Design review of the part built by this model. Coordinates are the model's own, in mm. A direction names the side the tool comes from. Give positions to 0.01 mm unless a question says otherwise; leave off trailing zeros. Order: outer loops, then holes, each group sorted by start corner. A loop starts at its lowest first (then second) coordinate and runs counter-clockwise, first axis right, second up. Notation, with made-up numbers: (8, 7) -> (48, 7) arc R21 ccw to (48, 23) -> close; hole circle Ø1 at (61.5, -37). An arc over 180 degrees is marked (long way). Answer in a Markdown table with one row per item. Add a question column.
```python
from build123d import *

# Parameters (mm, degrees)
SKETCH1_W           = 7.25
SKETCH1_H           = 20
SKETCH1_R           = 6
BOSS_EXTRUDE1_DEPTH = 40
SKETCH2_W           = 42
SKETCH2_H           = 22
CUT_EXTRUDE1_DEPTH  = 25
SKETCH3_R           = 2
CUT_EXTRUDE2_DEPTH  = 12
SKETCH4_R           = 9.5
CUT_EXTRUDE3_DEPTH  = 5
SKETCH5_R           = 9.5
CUT_EXTRUDE4_DEPTH  = 6
SKETCH7_W           = 7
SKETCH7_H           = 2
SKETCH7_H_2         = 1.8
CUT_EXTRUDE5_DEPTH  = 2.4
BOSS_EXTRUDE2_REACH = 75.701
SKETCH9_R           = 13.5
SKETCH9_R_2         = 10.05
BOSS_EXTRUDE3_REACH = 50.701
SKETCH10_R          = 10.05
SKETCH11_R          = 1.9
CUT_EXTRUDE7_DEPTH  = 13.5


with BuildPart() as part:
    # Sketch1 → Boss-Extrude1 (new body)
    with BuildSketch(Plane(origin=(0, 0, 0), x_dir=(1, 0, 0), z_dir=(0, 1, 0))):
        with BuildLine():
            Line((-30.25, -10), (-37.5, -10))
            Line((-37.5, -10), (-37.5, 10))
            Line((-37.5, 10), (-30.25, 10))
            Line((-30.25, 10), (-18.466185313, 10))
            ThreePointArc((-18.466185313, 10), (-13.083157843, 16.426532831), (-5.61521172, 20.235350191))
            Line((-5.61521172, 20.235350191), (-42.5, 10))
            Line((-42.5, 10), (-42.5, -10))
            Line((-42.5, -10), (-5.61521172, -20.235350191))
            ThreePointArc((-5.61521172, -20.235350191), (-13.083157843, -16.426532831), (-18.466185313, -10))
            Line((-18.466185313, -10), (-30.25, -10))
        make_face()
        with Locations((-33.875, 0)):
            Rectangle(SKETCH1_W, SKETCH1_H)
        with BuildLine():
            ThreePointArc((-18.466185313, 10), (-21, 0), (-18.466185313, -10))
            Line((-18.466185313, -10), (9.75, -10))
            Line((9.75, -10), (9.75, 10))
            Line((9.75, 10), (-18.466185313, 10))
        make_face()
        Circle(SKETCH1_R, mode=Mode.SUBTRACT)
        with BuildLine():
            Line((-30.25, 10), (-30.25, -10))
            Line((-30.25, -10), (-18.466185313, -10))
            ThreePointArc((-18.466185313, -10), (-21, 0), (-18.466185313, 10))
            Line((-18.466185313, 10), (-30.25, 10))
        make_face()
        with BuildLine():
            Line((9.75, -10), (-18.466185313, -10))
            ThreePointArc((-18.466185313, -10), (-13.083157843, -16.426532831), (-5.61521172, -20.235350191))
            ThreePointArc((-5.61521172, -20.235350191), (12.709849603, -16.717048874), (21, 0))
            ThreePointArc((21, 0), (12.709849603, 16.717048874), (-5.61521172, 20.235350191))
            ThreePointArc((-5.61521172, 20.235350191), (-13.083157843, 16.426532831), (-18.466185313, 10))
            Line((-18.466185313, 10), (9.75, 10))
            Line((9.75, 10), (17, 10))
            Line((17, 10), (17, -10))
            Line((17, -10), (9.75, -10))
        make_face()
        with Locations((13.375, 0)):
            Rectangle(SKETCH1_W, SKETCH1_H)
    extrude(amount=BOSS_EXTRUDE1_DEPTH)

    # Sketch2 → Cut-Extrude1 (cut)
    with BuildSketch(Plane(origin=(0, 40, 0), x_dir=(1, 0, 0), z_dir=(0, 1, 0))):
        with Locations((-10, 0)):
            Rectangle(SKETCH2_W, SKETCH2_H)
    extrude(amount=-CUT_EXTRUDE1_DEPTH, mode=Mode.SUBTRACT)

    # Sketch3 → Cut-Extrude2 (cut)
    with BuildSketch(Plane(origin=(0, 40, 0), x_dir=(1, 0, 0), z_dir=(0, 1, 0))):
        with Locations((14.75, 5)):
            Circle(SKETCH3_R)
        with Locations((14.75, -5)):
            Circle(SKETCH3_R)
        with Locations((-34.75, 5)):
            Circle(SKETCH3_R)
        with Locations((-34.75, -5)):
            Circle(SKETCH3_R)
    extrude(amount=-CUT_EXTRUDE2_DEPTH, mode=Mode.SUBTRACT)

    # Sketch4 → Cut-Extrude3 (cut)
    with BuildSketch(Plane(origin=(0, 15, 0), x_dir=(1, 0, 0), z_dir=(0, 1, 0))):
        Circle(SKETCH4_R)
    extrude(amount=-CUT_EXTRUDE3_DEPTH, mode=Mode.SUBTRACT)

    # Sketch5 → Cut-Extrude4 (cut)
    with BuildSketch(Plane.XZ):
        Circle(SKETCH5_R)
    extrude(amount=-CUT_EXTRUDE4_DEPTH, mode=Mode.SUBTRACT)

    # Sketch7 → Cut-Extrude5 (cut)
    with BuildSketch(Plane(origin=(0, 40, 0), x_dir=(1, 0, 0), z_dir=(0, 1, 0))):
        with Locations((-34.5, 0)):
            Rectangle(SKETCH7_W, SKETCH7_H)
        with Locations((14.5, 0)):
            Rectangle(SKETCH7_W, SKETCH7_H_2)
    extrude(amount=-CUT_EXTRUDE5_DEPTH, mode=Mode.SUBTRACT)

    # Sketch9 → Boss-Extrude2 (add, up to next)
    with BuildSketch(Plane(origin=(-8.961867673, -4.60437291, 43.807681948), x_dir=(0, 0.994521895, 0.104528463), z_dir=(0.199367934, 0.102430023, -0.974556575)), mode=Mode.PRIVATE) as boss_extrude2_sk1:
        with Locations((22.005607966, -1.9070974)):
            Circle(SKETCH9_R)
        with Locations((22.005607966, -1.9070974)):
            Circle(SKETCH9_R_2, mode=Mode.SUBTRACT)
    boss_extrude2_tool1 = extrude(boss_extrude2_sk1.sketch, amount=BOSS_EXTRUDE2_REACH, mode=Mode.PRIVATE) - part.part
    add(boss_extrude2_tool1.solids().sort_by_distance((-10.83068, 4.27413, 44.358542))[0])

    # Sketch10 → Boss-Extrude3 (add, up to next)
    with BuildSketch(Plane(origin=(-3.977669313, -2.043622323, 19.443767584), x_dir=(0.979924705, -0.020839624, 0.198275776), z_dir=(-0.199367934, -0.102430023, 0.974556575)), mode=Mode.PRIVATE) as boss_extrude3_sk1:
        with Locations((-1.9070974, 22.005607966)):
            Circle(SKETCH10_R)
    boss_extrude3_tool1 = extrude(boss_extrude3_sk1.sketch, amount=-BOSS_EXTRUDE3_REACH, mode=Mode.PRIVATE) - part.part
    add(boss_extrude3_tool1.solids().sort_by_distance((-5.846481, 19.88118, 21.365849))[0])

    # Sketch11 → Cut-Extrude7 (cut, symmetric)
    with BuildSketch(Plane(origin=(-1.868811857, 0.039743192, -0.378131217), x_dir=(-0.199367934, -0.102430023, 0.974556575), z_dir=(-0.979924705, 0.020839624, -0.198275776))):
        with Locations((32.45139953, 22.005607966)):
            Circle(SKETCH11_R)
    extrude(amount=CUT_EXTRUDE7_DEPTH, both=True, mode=Mode.SUBTRACT)


solid = part.part
```
1) Add section C-C, the plane z = 5. Write out the cut boundary in (x, y).
2) Machinability: for faces 3 (the face through (-5.984, 20.024, 21.353)), 4 (the face through (4.38, 2.96, -8.43)), 5 (the face through (-15, 15, 0)), which of the approach directions +Z, -Z, +X, -X, +Y, -Y give a long, thin tool a straight path to every point of the face, cutting with its end or side? Answer none if there is none.
3) For L1, parallel to Z at x = -34.75, y = 31; L2, parallel to X at y = 34.5, z = 3.5; L3, parallel to Z at x = 14.75, y = 34.75, list the stretches that pass through material, from the lowest coordinate up.
4) Add section A-A, the plane y = 36.5. Write out the cut boundary in (x, z), and give its area (3 significant figures).
5) Mouldability with a two-part tool opening along Z and no side actions: class faces 1 (the face through (15, 28, -5)), 2 (the face through (-11, 40, 14)) as +Z half, -Z half, draft (parallel to the pull), parting line (faces both ways), or undercut.
6) Clearance check with flat-ended pins moving along their axes: P1, Ø21, axis at x = 2, z = 3, coming from the -Y side; P2, Ø5.5, axis at x = -1, z = -0.5, coming from the +Y side; P3, Ø1.2, axis at x = 15.5, z = -5.5, coming from the +Y side; P4, Ø2.5, axis at x = 16, y = 38.5, coming from the -Z side. State where each tip first meets the part, or that it passes through.
7) Add section B-B, the plane x = -29. Write out the cut boundary in (y, z).
8) Add section D-D, the plane x = 0. Give the number of separate pieces and of enclosed holes in the cut face, and give its area (3 significant figures).
Verdict:
| question | item | result |
|---|---|---|
| 1 | outline | (-42.5, 0) -> (-8.08, 0) -> (-8.08, 6) -> (-3.32, 6) -> (-3.32, 10) -> (-8.08, 10) -> (-8.08, 15) -> (-31, 15) -> (-31, 40) -> (-32.75, 40) -> (-32.75, 28) -> (-36.75, 28) -> (-36.75, 40) -> (-42.5, 40) -> close; (3.32, 6) -> (8.08, 6) -> (8.08, 0) -> (20.4, 0) -> (20.4, 40) -> (16.75, 40) -> (16.75, 28) -> (12.75, 28) -> (12.75, 40) -> (11, 40) -> (11, 15) -> (8.08, 15) -> (8.08, 10) -> (3.32, 10) -> close |
| 2 | face 3 | none |
| 2 | face 4 | -Y |
| 2 | face 5 | +Y |
| 3 | L1 | z = -12.15 to -7, -3 to 3, 7 to 12.15 |
| 3 | L2 | x = -42.5 to -36.07, -33.43 to -31, 11 to 13.43, 16.07 to 20.71 |
| 3 | L3 | z = -14.95 to -7, -3 to 3, 7 to 14.95 |
| 4 | outline | (-42.5, -10) -> (-5.62, -20.24) arc R21 ccw (long way) to (-5.62, 20.24) -> (-42.5, 10) -> close; hole circle Ø4 at (-34.75, -5); hole circle Ø4 at (-34.75, 5); hole (-31, -11) -> (11, -11) -> (11, 11) -> (-31, 11) -> close; hole circle Ø4 at (14.75, -5); hole circle Ø4 at (14.75, 5) |
| 4 | area | 1,070 mm2 |
| 5 | face 1 | undercut |
| 5 | face 2 | draft |
| 6 | P1 | stops at y = 0 |
| 6 | P2 | passes through |
| 6 | P3 | stops at y = 28 |
| 6 | P4 | stops at z = -14.95 |
| 7 | outline | (0, -13.75) -> (40, -13.75) -> (40, -11) -> (15, -11) -> (15, 11) -> (40, 11) -> (40, 13.75) -> (0, 13.75) -> close |
| 8 | separate pieces | 2 |
| 8 | enclosed holes | 1 |
| 8 | area | 1,210 mm2 |
